Solid Edge part; units mm, degrees
sketch "Sketch1" plane through (0, 0, 0) normal (0, 0, 1) x (1, 0, 0)
  line L0 (12.5, -27.96) -> (12.5, 27.96)
  line L1 (12.5, 27.96) -> (-12.5, 27.96)
  line L2 (-12.5, 27.96) -> (-12.5, -27.96)
  line L3 (-12.5, -27.96) -> (12.5, -27.96)
extrude "Protrusion1" add sketch "Sketch1" against normal blind 1.5
sketch "Sketch2" plane through (0, 0, -1.5) normal (0, 0, -1) x (0, 1, 0)
  line L0 (-26.46, 11) -> (26.46, 11)
  line L1 (26.46, 11) -> (26.46, -11)
  line L2 (26.46, -11) -> (-26.46, -11)
  line L3 (-26.46, -11) -> (-27.96, -11)
  line L4 (-27.96, -11) -> (-27.96, -12.5)
  line L5 (27.96, -12.5) -> (-27.96, -12.5)
  line L6 (27.96, 12.5) -> (27.96, -12.5)
  line L7 (-27.96, 12.5) -> (27.96, 12.5)
  line L8 (-27.96, 11) -> (-27.96, 12.5)
  line L9 (-26.46, 11) -> (-27.96, 11)
extrude "ExtrudedProtrusion_2" add sketch "Sketch2" along normal blind 3
sketch "Sketch3" plane through (0, -0.75, -1.5) normal (0, 0, -1) x (-1, 0, 0)
  circle A0 centre (4.6516, 20.9885) radius 1.5011
  circle A1 centre (-4.85, 20.9885) radius 1.5
extrude "Cutout1" cut sketch "Sketch3" against normal up to vertex (1.5 mm away)
fillet "Round_1" radius 0.75 12 edges at (12.5, -27.96, -2.25) (-12.5, -27.96, -2.25) (-12.5, 0, 0) (0, -27.96, 0) (-11, -27.96, -3) (11, -27.96, -3) (-12.5, 27.96, -2.25) (0, 27.96, 0) (12.5, 0, 0) (12.5, 0, -4.5) (12.5, 27.96, -2.25) (0, 27.96, -4.5)
fillet "Round_2" radius 3 2 edges at (-11, 26.46, -3) (11, 26.46, -3)
properties material "ABS Plastic, medium impact"
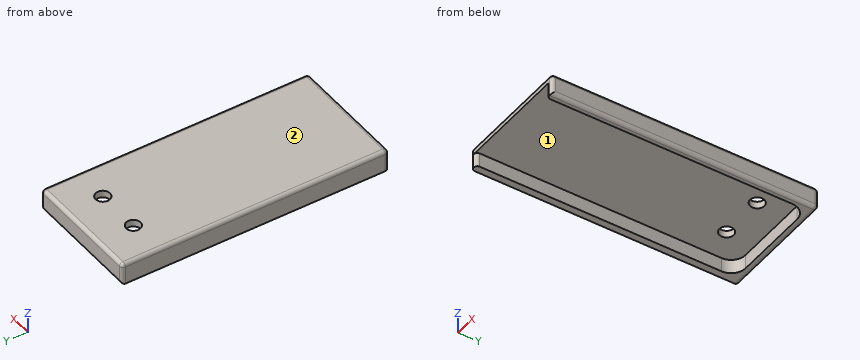
The listing builds one solid part. Answer for the finished solid, in the listing's coordinates (mm). Face numbers are marked on the shaded views. A direction names the side the tool comes from. Give positions to 0.01 mm unless a question says otherwise; leave off trailing zeros. Write each loop counter-clockwise with the first axis right and the second up, starting at its lowest first coordinate (ties: lowest second). Pieces come first, ordered by that corner, then holes.
1) A tool of negligible diameter and unlimited length cuts with its end or side. For the marked faces 1 and 2, from which of +Z, -Z, +X, -X, +Y, -Y can it reach the whole face along a straight path? Write none if from no direction.
2) Section C-C (y = 19.5) is taken. Write down the section's boundary in (x, z), and give its area (3 significant figures).
3) Find the intervals of material crossed by L1, parallel to X at y = -11.5, z = -1.95; L2, parallel to Y at x = 4.85, z = -0.65; L3, parallel to Z at x = 8, y = -11, in increasing order.
4) Section D-D (y = 6) is taken. Write down the section's boundary in (x, z), and give its area (3 significant figures).
5) Section A-A (x = 4.85) is taken. Write down the section's boundary in (y, z).
6) Given P1, Ø4, axis at x = 5, y = -2, coming from the -Z side; P2, Ø1.8, axis at x = -4.65, y = 20.24, coming from the +Z side; P3, Ø0.9, axis at x = 4, z = -2.5, coming from the -Y side, each flat-ended and moving along its own axis, determine where each tip first touches the part or whether it passes through.
Response:
1. face 1: -Z, -Y
1. face 2: +Z, +X, -X, +Y, -Y
2. outline: (-12.5, -4.5) - (-11, -4.5) - (-11, -1.5) - (-5.96, -1.5) - (-5.96, 0) - (-11.75, 0) arc R0.75 ccw to (-12.5, -0.75) - close; (-3.34, -1.5) - (3.54, -1.5) - (3.54, 0) - (-3.34, 0) - close; (6.16, -1.5) - (11, -1.5) - (11, -4.5) - (11.75, -4.5) arc R0.75 ccw to (12.5, -3.75) - (12.5, -0.75) arc R0.75 ccw to (11.75, 0) - (6.16, 0) - close
2. area: 38.3 mm2
3. L1: x = -12.5 to -11, 11 to 12.5
3. L2: y = -27.95 to 18.74, 21.74 to 27.95
3. L3: z = -1.5 to 0
4. outline: (-12.5, -4.5) - (-11, -4.5) - (-11, -1.5) - (11, -1.5) - (11, -4.5) - (11.75, -4.5) arc R0.75 ccw to (12.5, -3.75) - (12.5, -0.75) arc R0.75 ccw to (11.75, 0) - (-11.75, 0) arc R0.75 ccw to (-12.5, -0.75) - close
4. area: 46.1 mm2
5. outline: (-27.96, -1.5) - (18.74, -1.5) - (18.74, 0) - (-27.21, 0) arc R0.75 ccw to (-27.96, -0.75) - close; (21.74, -1.5) - (26.46, -1.5) - (26.46, -4.5) - (27.21, -4.5) arc R0.75 ccw to (27.96, -3.75) - (27.96, -0.75) arc R0.75 ccw to (27.21, 0) - (21.74, 0) - close
6. P1: stops at z = -1.5
6. P2: passes through
6. P3: stops at y = 26.46
